from build123d import *

# Parameters (mm, degrees)
SKETCH_R        = 9
PAD_DEPTH       = 20
SKETCH001_W     = 6
SKETCH001_H     = 13.2
POCKET_DEPTH    = 10
SKETCH002_R     = 1.6
POCKET001_DEPTH = 11
FILLET_R        = 3
SKETCH003_R     = 2.5
POCKET002_DEPTH = 3
SKETCH004_R     = 1.1
POCKET003_DEPTH = 13


with BuildPart() as part:
    # Sketch → Pad (new body)
    with BuildSketch(Plane.XY):
        Circle(SKETCH_R)
    extrude(amount=PAD_DEPTH)

    # Sketch001 (on Face2 of Pad) → Pocket (cut)
    with BuildSketch(Plane(origin=(0, 0, 0), x_dir=(1, 0, 0), z_dir=(0, 0, -1))):
        with Locations((0, -1.063468)):
            Rectangle(SKETCH001_W, SKETCH001_H)
    extrude(amount=-POCKET_DEPTH, mode=Mode.SUBTRACT)

    # Sketch002 (on Face3 of Pocket) → Pocket001 (cut)
    with BuildSketch(Plane.XY.offset(20)):
        with Locations((0, 4)):
            Circle(SKETCH002_R)
    extrude(amount=-POCKET001_DEPTH, mode=Mode.SUBTRACT)

    # Fillet
    fillet_edges = [part.edges().sort_by_distance(p)[0] for p in [
        (-9, 0, 20),
    ]]
    fillet(fillet_edges, radius=FILLET_R)

    # Sketch003 (on Face10 of Fillet) → Pocket002 (cut)
    with BuildSketch(Plane(origin=(0, 0, 10), x_dir=(1, 0, 0), z_dir=(0, 0, -1))):
        with Locations((0, -4)):
            Circle(SKETCH003_R)
    extrude(amount=-POCKET002_DEPTH, mode=Mode.SUBTRACT)

    # Sketch004 (on Face6 of Pocket002) → Pocket003 (cut)
    with BuildSketch(Plane(origin=(3, 0, 0), x_dir=(0, -1, 0), z_dir=(-1, 0, 0))):
        with Locations((2.337519, 1.3)):
            Circle(SKETCH004_R)
        with Locations((-4.657478, 1.3)):
            Circle(SKETCH004_R)
    extrude(amount=-POCKET003_DEPTH, mode=Mode.SUBTRACT)


solid = part.part
The model under review builds one solid part; all positions refer to its coordinate system, in mm. A direction names the side the tool comes from. Give positions to 0.01 mm unless a question says otherwise; leave off trailing zeros. Write each loop counter-clockwise with the first axis right and the second up, starting at its lowest first coordinate (ties: lowest second). Pieces come first, ordered by that corner, then holes. Notation, with made-up numbers: M -22.75,39.25 L 1.25,39.25 A22 cw 1.25,74.25 Z; hole C 71,26 d7. An arc over 180 degrees is marked long. One line per question, with ' | ' between items. Start each with the question number.
Item 1: We need section C-C on y = 4. Give the number of separate pieces and of enclosed holes in the cut face, plus the area to 3 significant figures.
Item 2: We need section D-D on z = 15. Write out the cut boundary in (x, y).
Item 3: We need section B-B on z = 1.3. Write out the cut boundary in (x, y).
Item 4: We need section A-A on x = 0. Write out the cut boundary in (y, z).
Item 5: Wall thickness on line 1 (Y direction, x = 0, z = 11.45); line 2 (Y direction, x = 0, z = 15); line 3 (Z direction, x = 0, y = -2.25): over which ranges is each line inside the solid? List them lowest first. Write a range as from..to.
Item 6: For faces 1 (the cylindrical face through (5.92, -1.24, 1.35)), 2 (the flat face through (0, 0, 20)), 3 (the cylindrical face through (-0.33, 1.52, 11.48)), list the 3-axis set-ups (+Z, -Z, +X, -X, +Y, -Y) from which the entire face can be reached by the end or side of a thin tool; tool diameter is ignored.
Item 7: Draft analysis for pull direction X (two halves, no side actions). For faces 4 (the flat face through (-3, 1, 5)), 5 (the flat face through (4, 0, 0)), 6 (the cylindrical face through (-1.172, 8.923, 8.381)), state which applies: released by +X, released by -X, zero draft, split by the parting line, or undercut.
Item 8: For pin 1 (2 mm diameter, centred on y = 4.5, z = 8, fed in from -X); pin 2 (6 mm diameter, centred on x = 7, z = 6, fed in from -Y); pin 3 (3 mm diameter, centred on x = -1.5, z = 5.5, fed in from -Y); pin 4 (5 mm diameter, centred on x = -3, z = 13, fed in from +Y), all flat-tipped, find the tip position at first contact; note any pin that passes through.
Results found:
1) separate pieces: 3 | enclosed holes: 0 | area: 212 mm2
2) outline: C 0,0 d18; hole C 0,4 d3.2
3) outline: M -3,-5.54 L -3,7.66 L 3,7.66 L 3,5.76 L 6.92,5.76 A9 ccw long 8.32,-3.44 L 3,-3.44 L 3,-5.54 Z; M 3,-1.24 L 8.91,-1.24 A9 ccw 8.27,3.56 L 3,3.56 Z
4) outline: M -9,0 L -5.54,0 L -5.54,10 L 1.5,10 L 1.5,13 L 2.4,13 L 2.4,20 L -6,20 A3 ccw -9,17 Z; M 5.6,13 L 6.5,13 L 6.5,10 L 7.66,10 L 7.66,0 L 9,0 L 9,17 A3 ccw 6,20 L 5.6,20 Z
5) line 1: y = -9..1.5, 6.5..9 | line 2: y = -9..2.4, 5.6..9 | line 3: z = 10..20
6) face 1: +X | face 2: +Z, +X, -X, +Y, -Y | face 3: -Z
7) face 4: undercut | face 5: zero draft | face 6: split by the parting line
8) pin 1: stops at x = -8.29 | pin 2: stops at y = -8.06 | pin 3: stops at y = -9 | pin 4: stops at y = 8.99
